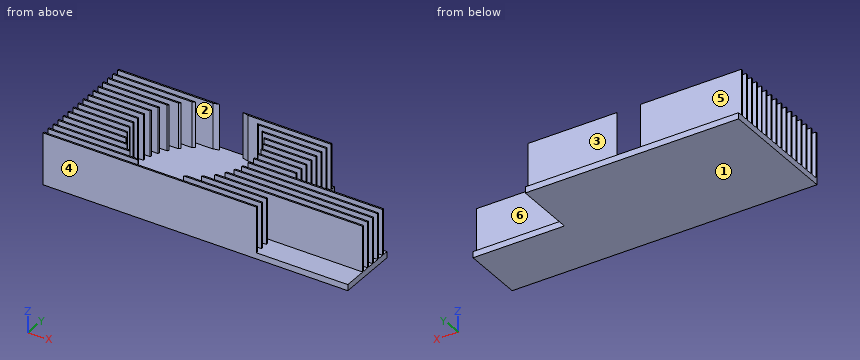
from build123d import *

# Parameters (mm, degrees)
MAIN_SKETCH_W              = 100
MAIN_SKETCH_H              = 40
MAIN_DEPTH                 = 2
ESQUISSE2_W                = 100
ESQUISSE2_H                = 0.5
BOSS_EXTRU_2_DEPTH         = 15
R_P_TITION_LIN_AIRE2_COUNT = 16
R_P_TITION_LIN_AIRE2_PITCH = 2.54
ESQUISSE3_W                = 30
ESQUISSE3_H                = 7.5
ENL_V_MAT_EXTRU_1_DEPTH    = 16
ESQUISSE4_W                = 30
ESQUISSE4_H                = 20
ENL_V_MAT_EXTRU_2_DEPTH    = 25
ESQUISSE5_R                = 19
ENL_V_MAT_EXTRU_3_DEPTH    = 16


with BuildPart() as part:
    # Main-Sketch → Main (new body)
    with BuildSketch(Plane.XY):
        with Locations((50, 20)):
            Rectangle(MAIN_SKETCH_W, MAIN_SKETCH_H)
    extrude(amount=MAIN_DEPTH)

    # Esquisse2 → Boss.-Extru.2 (add)
    with BuildSketch(Plane.XY.offset(2)):
        with Locations((50, 0.25)):
            Rectangle(ESQUISSE2_W, ESQUISSE2_H)
    boss_extru_2 = extrude(amount=BOSS_EXTRU_2_DEPTH)

    # Répétition linéaire2: Boss.-Extru.2 ×16
    with Locations(*[(0, i * R_P_TITION_LIN_AIRE2_PITCH, 0) for i in range(1, R_P_TITION_LIN_AIRE2_COUNT)]):
        add(boss_extru_2)

    # Esquisse3 → Enlèv. mat.-Extru.1 (cut, through all)
    with BuildSketch(Plane.XY.offset(2)):
        with Locations((85, 3.75)):
            Rectangle(ESQUISSE3_W, ESQUISSE3_H)
    extrude(amount=ENL_V_MAT_EXTRU_1_DEPTH, mode=Mode.SUBTRACT)

    # Esquisse4 → Enlèv. mat.-Extru.2 (cut, symmetric)
    with BuildSketch(Plane.XY.offset(2)):
        with Locations((85, 30)):
            Rectangle(ESQUISSE4_W, ESQUISSE4_H)
    extrude(amount=ENL_V_MAT_EXTRU_2_DEPTH, both=True, mode=Mode.SUBTRACT)

    # Esquisse5 → Enlèv. mat.-Extru.3 (cut, through all)
    with BuildSketch(Plane.XY.offset(2)):
        with Locations((37, 20)):
            Circle(ESQUISSE5_R)
    extrude(amount=ENL_V_MAT_EXTRU_3_DEPTH, mode=Mode.SUBTRACT)


solid = part.part
Source: CAD feature listing. Evaluate the final solid. Frame: model axes, mm. Face numbers are marked on the shaded views. A direction names the side the tool comes from. Round coordinates to 2 decimals unless told otherwise and drop trailing zeros. Loops run counter-clockwise (first coordinate to the right, second up) from the corner with the lowest first, then second, coordinate; pieces in that order, holes last. Notation, with made-up numbers: (-15.75, -34.75) -> (3.25, -34.75) arc R13 cw to (3.25, -13.75) -> close; hole circle Ø7 at (47.25, 75). An arc over 180 degrees is marked (long way). Answer as a JSON object with one key per item and string values. Group by question number.
Q1. Section query B-B (z = 10.25). State how many separate pieces and enclosed holes the cut face has, plus the area to 3 significant figures.
Q2. Section query A-A (x = 92.5). Output: boundary loops of the cut face in (y, z), plus the area to 3 significant figures.
Q3. Section query D-D (x = 34.5). Output: boundary loops of the cut face in (y, z).
Q4. Access query for the marked faces 4, 5 and 6. Directions: +Z, -Z, +X, -X, +Y, -Y. A direction counts if a zero-diameter tool reaches every point of the face in a straight line with its end or side. Return the directions, or none.
Q5. Mould query, pull axis Y, two halves, no side actions, for the marked faces 1, 2 and 3. Classes: pulls with the +Y half, pulls with the -Y half, needs draft (parallel to the pull), parting line crosses it, or undercut.
Q6. Section query C-C (y = 32). Output: boundary loops of the cut face in (x, z).
Q7. Contact query for flat-ended pins moving along their axis: P1, Ø5, axis at x = 21.5, z = 6, coming from the +Y side; P2, Ø10, axis at y = 25, z = 11.5, coming from the +X side; P3, Ø7.5, axis at x = 84.5, z = 9.5, coming from the +Y side. Output: stop coordinate, or through.
Q8. Ray query, line 1 (Y direction, x = 93, z = 8); line 2 (Z direction, x = 48, y = 35); line 3 (X direction, y = 13, z = 10). Return the intervals inside material, ascending. Write a range as from..to.
Completed:
{
 "1": {"separate pieces": "31", "enclosed holes": "0", "area": "411 mm²"},
 "2": {"outline": "(0, 0) -> (20, 0) -> (20, 2) -> (18.28, 2) -> (18.28, 17) -> (17.78, 17) -> (17.78, 2) -> (15.74, 2) -> (15.74, 17) -> (15.24, 17) -> (15.24, 2) -> (13.2, 2) -> (13.2, 17) -> (12.7, 17) -> (12.7, 2) -> (10.66, 2) -> (10.66, 17) -> (10.16, 17) -> (10.16, 2) -> (8.12, 2) -> (8.12, 17) -> (7.62, 17) -> (7.62, 2) -> (0, 2) -> close", "area": "77.5 mm²"},
 "3": {"outline": "(0, 0) -> (40, 0) -> (40, 2) -> (0.5, 2) -> (0.5, 17) -> (0, 17) -> close"},
 "4": {"face 4": "+Z, -Z, +X, -X, -Y", "face 5": "+Z, +X, -X, +Y", "face 6": "+Z, +X, -X"},
 "5": {"face 1": "needs draft", "face 2": "undercut", "face 3": "pulls with the +Y half"},
 "6": {"outline": "(0, 0) -> (70, 0) -> (70, 2) -> (0, 2) -> close"},
 "7": {"P1": "y = 38.6", "P2": "x = 70", "P3": "y = 18.28"},
 "8": {"line 1": "7.62..8.12, 10.16..10.66, 12.7..13.2, 15.24..15.74, 17.78..18.28", "line 2": "0..2", "line 3": "0..19.34, 54.66..100"}
}
